```python
from build123d import *

# Parameters (mm, degrees)
BOSS_EXTRUDE1_DEPTH  = 20
SKETCH2_W            = 45
SKETCH2_H            = 20
CUT_EXTRUDE1_DEPTH   = 20
FILLET1_R            = 9.75
FILLET1_OF_MIRROR4_R = 9.75


with BuildPart() as part:
    # Sketch1 → Boss-Extrude1 (new body)
    with BuildSketch(Plane(origin=(0, 0, 0), x_dir=(1, 0, 0), z_dir=(0, 1, 0))):
        with BuildLine():
            Line((22.360679775, 20), (75, 20))
            Line((75, 20), (75, -20))
            Line((75, -20), (22.360679775, -20))
            ThreePointArc((22.360679775, -20), (12.247448714, -27.386127875), (0, -30))
            Line((0, -30), (0, -20))
            Line((0, -20), (0, 20))
            Line((0, 20), (0, 30))
            ThreePointArc((0, 30), (12.247448714, 27.386127875), (22.360679775, 20))
        make_face()
    boss_extrude1 = extrude(amount=BOSS_EXTRUDE1_DEPTH)

    # Sketch2 → Cut-Extrude1 (cut)
    with BuildSketch(Plane(origin=(0, 20, 0), x_dir=(1, 0, 0), z_dir=(0, 1, 0))):
        with BuildLine():
            Line((0, 5), (0, -5))
            ThreePointArc((0, -5), (2.738612788, -4.183300133), (4.582575695, -2))
            Line((4.582575695, -2), (7.228416147, -2))
            ThreePointArc((7.228416147, -2), (7.5, 0), (7.228416147, 2))
            Line((7.228416147, 2), (4.582575695, 2))
            ThreePointArc((4.582575695, 2), (2.738612788, 4.183300133), (0, 5))
        make_face()
        with Locations((52.5, 0)):
            Rectangle(SKETCH2_W, SKETCH2_H)
    cut_extrude1 = extrude(amount=-CUT_EXTRUDE1_DEPTH, mode=Mode.SUBTRACT)

    # Fillet1
    fillet1_edges = [part.edges().sort_by_distance(p)[0] for p in [
        (75, 10, -20),
        (75, 10, 20),
    ]]
    fillet(fillet1_edges, radius=FILLET1_R)

    # Mirror4: Boss-Extrude1, Cut-Extrude1 across plane
    add(boss_extrude1.mirror(Plane(origin=(0, 0, 0), x_dir=(0, 0, 1), z_dir=(1, 0, 0))))
    add(cut_extrude1.mirror(Plane(origin=(0, 0, 0), x_dir=(0, 0, 1), z_dir=(1, 0, 0))), mode=Mode.SUBTRACT)

    # Fillet1 of Mirror4
    fillet1_of_mirror4_edges = [part.edges().sort_by_distance(p)[0] for p in [
        (-75, 10, -20),
        (-75, 10, 20),
    ]]
    fillet(fillet1_of_mirror4_edges, radius=FILLET1_OF_MIRROR4_R)


solid = part.part
```
Source: CAD feature listing. Evaluate the final solid. Frame: model axes, mm. A direction names the side the tool comes from. Coordinates: 2 decimals unless noted, no trailing zeros. Loops run counter-clockwise (first coordinate to the right, second up) from the corner with the lowest first, then second, coordinate; pieces in that order, holes last. Notation, with made-up numbers: M 13.5,30.25 L 19.5,30.25 A28 ccw 19.5,67.25 Z; hole C 77,-2.75 d9. An arc over 180 degrees is marked long. Put each result on its own line as item: value. Start each with the question number.
1) Contact query for flat-ended pins moving along their axis: pin 1 Ø6 at (x, y) = (-42.5, 12) entering from +Z; pin 2 Ø2 at (y, z) = (12.5, 19.5) entering from -X; pin 3 Ø10 at (y, z) = (7, 2.5) entering from +X. Output: stop coordinate, or through.
2) Pull-direction query (X, two-part tool) for faces 5 (the face through (7.5, 10.1, 0)), 6 (the face through (-30, 10, 0)), 7 (the face through (52, 10, -10)), 8 (the face through (6, 10, 2)); classes: pulls with the +X half, pulls with the -X half, needs draft (parallel to the pull), parting line crosses it, or undercut.
3) Cut plane A-A on x = 39. Return the cut outline in (y, z).
4) Ray query, L1, parallel to Z at x = 41, y = 7.25; L2, parallel to Z at x = 29, y = 7.75; L3, parallel to X at y = 18, z = 8. Return the intervals inside material, ascending. Write a range as from..to.
5) Cut plane C-C on z = -22. Return the cut outline in (x, y), then the cut area to 3 significant figures.
6) Cut plane D-D on x = -12. Return the cut outline in (y, z), then the cut area to 3 significant figures.
7) Reachability of faces 1 (the face through (-44, 10, -20)), 2 (the face through (52, 10, 10)), 3 (the face through (-7.5, 10.1, 0)), 4 (the face through (44, 10, -20)) from +Z, -Z, +X, -X, +Y, -Y: full face, straight path, thin tool, end or side. Return the list, or none.
8) Cut plane B-B on y = 7.5. Return the cut outline in (x, z), then the cut area to 3 significant figures.
The answers:
1. pin 1: stops at z = 20
1. pin 2: stops at x = -70.45
1. pin 3: stops at x = 30
2. face 5: undercut
2. face 6: pulls with the -X half
2. face 7: needs draft
2. face 8: undercut
3. outline: M 0,-20 L 20,-20 L 20,-10 L 0,-10 Z; M 0,10 L 20,10 L 20,20 L 0,20 Z
4. L1: z = -20..-10, 10..20
4. L2: z = -20..20
4. L3: x = -30..30
5. outline: M -20.4,0 L 20.4,0 L 20.4,20 L -20.4,20 Z
5. area: 816 mm²
6. outline: M 0,-27.5 L 20,-27.5 L 20,27.5 L 0,27.5 Z
6. area: 1,100 mm²
7. face 1: -Z, -X, +Y, -Y
7. face 2: +X, +Y, -Y
7. face 3: +Y, -Y
7. face 4: -Z, +X, +Y, -Y
8. outline: M -75,-10.25 A9.75 ccw -65.25,-20 L -22.36,-20 A30 ccw 22.36,-20 L 65.25,-20 A9.75 ccw 75,-10.25 L 75,-10 L 30,-10 L 30,10 L 75,10 L 75,10.25 A9.75 ccw 65.25,20 L 22.36,20 A30 ccw -22.36,20 L -65.25,20 A9.75 ccw -75,10.25 L -75,10 L -30,10 L -30,-10 L -75,-10 Z; hole M -7.23,-2 L -4.58,-2 A5 ccw 4.58,-2 L 7.23,-2 A7.5 ccw 7.23,2 L 4.58,2 A5 ccw -4.58,2 L -7.23,2 A7.5 ccw Z
8. area: 4,640 mm²
